The listing builds one solid part. Answer for the finished solid, in the listing's coordinates (mm). A direction names the side the tool comes from. Round coordinates to 2 decimals unless told otherwise and drop trailing zeros. Order: outer loops, then holes, each group sorted by start corner. A loop starts at its lowest first (then second) coordinate and runs counter-clockwise, first axis right, second up. Notation, with made-up numbers: (-37.5, -22) - (4.5, -22) arc R15 cw to (4.5, -1) - close; hole circle Ø1 at (-29.75, 29.25). An arc over 180 degrees is marked (long way). Write item = value, one per line.
from build123d import *

# Parameters (mm, degrees)
SKETCH_3_R      = 1
EXTRUDE_3_DEPTH = 5


with BuildPart() as part:
    # 草图3 → 凸台-拉伸3 (new body)
    with BuildSketch(Plane.XY):
        with BuildLine():
            Line((2726.161531979, 4664.634627263), (2573.661531979, 4664.653356317))
            Line((2573.661531979, 4664.653356317), (2573.661531979, 4671.643884914))
            Line((2573.661531979, 4671.643884914), (2562.161531979, 4671.643884914))
            Line((2562.161531979, 4671.643884914), (2562.161531979, 4662.034400913))
            Line((2562.161531979, 4662.034400913), (2567.161531979, 4662.034400913))
            ThreePointArc((2567.161531979, 4662.034400913), (2568.661531979, 4663.534400913), (2570.161531979, 4662.034400913))
            Line((2570.161531979, 4662.034400913), (2570.161531979, 4659.234400913))
            ThreePointArc((2570.161531979, 4659.234400913), (2568.661531979, 4657.734400913), (2567.161531979, 4659.234400913))
            Line((2567.161531979, 4659.234400913), (2562.161531979, 4659.234400913))
            Line((2562.161531979, 4659.234400913), (2562.161531979, 4649.791778919))
            Line((2562.161531979, 4649.791778919), (2562.161531979, 4649.643884914))
            Line((2562.161531979, 4649.643884914), (2573.661531979, 4649.643884914))
            Line((2573.661531979, 4649.643884914), (2573.661531979, 4656.634400913))
            Line((2573.661531979, 4656.634400913), (2726.161531979, 4656.634400913))
            Line((2726.161531979, 4656.634400913), (2726.161531979, 4664.634627263))
        make_face()
        with Locations((2594.161531979, 4660.639111823)):
            Circle(SKETCH_3_R, mode=Mode.SUBTRACT)
        with Locations((2625.161531979, 4660.639111823)):
            Circle(SKETCH_3_R, mode=Mode.SUBTRACT)
        with Locations((2675.161531979, 4660.639111823)):
            Circle(SKETCH_3_R, mode=Mode.SUBTRACT)
    extrude(amount=EXTRUDE_3_DEPTH)


solid = part.part
Q1. Section A-A on z = 4 is taken. Determine the outline of the cut face in (x, y), then the cut area to 3 significant figures.
Model answer:
outline = (2562.16, 4649.64) - (2573.66, 4649.64) - (2573.66, 4656.63) - (2726.16, 4656.63) - (2726.16, 4664.63) - (2573.66, 4664.65) - (2573.66, 4671.64) - (2562.16, 4671.64) - (2562.16, 4662.03) - (2567.16, 4662.03) arc R1.5 cw to (2570.16, 4662.03) - (2570.16, 4659.23) arc R1.5 cw to (2567.16, 4659.23) - (2562.16, 4659.23) - close; hole circle Ø2 at (2594.16, 4660.64); hole circle Ø2 at (2625.16, 4660.64); hole circle Ø2 at (2675.16, 4660.64)
area = 1,440 mm^2
Q2. Find the intervals of material crossed by line 1 (X direction, y = 4664.75, z = 1.15); line 2 (Y direction, x = 2649, z = 3.6); line 3 (X direction, y = 4659.5, z = 3.35), in increasing order. Write a range as from..to.
Model answer:
line_1 = 2562.16..2573.66
line_2 = 4656.63..4664.64
line_3 = 2570.16..2726.16
Q3. Section C-C on x = 2636 is taken. Determine the outline of the cut face in (y, z).
Model answer:
outline = (4656.63, 0) - (4664.65, 0) - (4664.65, 5) - (4656.63, 5) - close
Q4. Section B-B on y = 4651.25 is taken. Determine the outline of the cut face in (x, z), then the cut area to 3 significant figures.
Model answer:
outline = (2562.16, 0) - (2573.66, 0) - (2573.66, 5) - (2562.16, 5) - close
area = 57.5 mm^2
Q5. Determine the mould class of faces 1 (the face through (2649, 4656.634, 2)), 2 (the face through (2565, 4659.234, 2)), 3 (the face through (2565, 4662.034, 2)), 4 (the face through (2625, 4663, 5)) for opening direction Y: released by +Y, released by -Y, zero draft, split by the parting line, or undercut.
Model answer:
face_1 = released by -Y
face_2 = undercut
face_3 = undercut
face_4 = zero draft
Q6. Flat-ended cylindrical pins translate along their axes: P1, Ø3, axis at x = 2699, z = 2.5, coming from the +Y side; P2, Ø1.5, axis at y = 4669.5, z = 2.5, coming from the +X side; P3, Ø2, axis at y = 4660.5, z = 1.5, coming from the -X side. Find the tip coordinate at first contact, or state that the pin passes through.
Model answer:
P1 = 4664.64
P2 = 2573.66
P3 = 2570.16
Q7. For faces 5 (the face through (2573.662, 4653, 2)), 6 (the face through (2568.695, 4657.735, 2.465)), 7 (the face through (2573.662, 4668, 2)), determine the directions among +Z, -Z, +X, -X, +Y, -Y from which every point of the face is accessible in a straight line to the end or side of a thin tool.
Model answer:
face_5 = +Z, -Z, +X, -Y
face_6 = +Z, -Z
face_7 = +Z, -Z, +X, +Y
